```python
from build123d import *

# Parameters (mm, degrees)
F0_R     = 5.5
F0_R_2   = 8
F1_DEPTH = 6
F3_DEPTH = 25
F4_W     = 30
F4_H     = 6
F5_DEPTH = 25
F6_W     = 21
F6_H     = 7
F6_H_2   = 6
F7_DEPTH = 25


with BuildPart() as f1:
    # F0 (on Front) → F1 (new body)
    with BuildSketch(Plane.XZ):
        with BuildLine():
            Line((-59.436191, 0), (-59.436191, -101.490244))
            Line((-59.436191, -101.490244), (-19.436191, -101.490244))
            Line((-19.436191, -101.490244), (-19.436191, -78.490244))
            ThreePointArc((-19.436191, -78.490244), (-16.507259, -71.419176), (-9.436191, -68.490244))
            Line((-9.436191, -68.490244), (0.563809, -68.490244))
            ThreePointArc((0.563809, -68.490244), (7.634877, -65.561312), (10.563809, -58.490244))
            Line((10.563809, -58.490244), (10.563809, -53.490244))
            Line((10.563809, -53.490244), (10.563809, -48.490244))
            ThreePointArc((10.563809, -48.490244), (7.634877, -41.419176), (0.563809, -38.490244))
            Line((0.563809, -38.490244), (-4.436191, -38.490244))
            Line((-4.436191, -38.490244), (-9.436191, -38.490244))
            ThreePointArc((-9.436191, -38.490244), (-16.507259, -35.561312), (-19.436191, -28.490244))
            Line((-19.436191, -28.490244), (-19.436191, 3.509756))
            ThreePointArc((-19.436191, 3.509756), (-16.507259, 10.580824), (-9.436191, 13.509756))
            ThreePointArc((-9.436191, 13.509756), (-2.365123, 16.438688), (0.563809, 23.509756))
            Line((0.563809, 23.509756), (0.563809, 33.509756))
            Line((0.563809, 33.509756), (0.563809, 43.509756))
            ThreePointArc((0.563809, 43.509756), (-2.365123, 50.580824), (-9.436191, 53.509756))
            ThreePointArc((-9.436191, 53.509756), (-43.651687, 40.011908), (-59.436191, 6.789303))
            Line((-59.436191, 6.789303), (-59.436191, 0))
        make_face()
        with Locations((-4.436191, -53.490244)):
            Circle(F0_R, mode=Mode.SUBTRACT)
        with Locations((-19.436191, 33.509756)):
            Circle(F0_R_2, mode=Mode.SUBTRACT)
    extrude(amount=F1_DEPTH)

    # F2 (on face) → F3 (cut)
    with BuildSketch(Plane.XZ.offset(6)):
        with BuildLine():
            Line((-59.436191, 6.789303), (-59.436191, -101.490244))
            Line((-59.436191, -101.490244), (-49.436191, -101.490244))
            Line((-49.436191, -101.490244), (-49.436191, 33.586102))
            ThreePointArc((-49.436191, 33.586102), (-56.388476, 20.916254), (-59.436191, 6.789303))
        make_face()
    extrude(amount=-F3_DEPTH, mode=Mode.SUBTRACT)

    # F4 (on face) → F5 (cut)
    with BuildSketch(Plane.XZ.offset(6)):
        with Locations((-34.436191, -98.490244)):
            Rectangle(F4_W, F4_H)
    extrude(amount=-F5_DEPTH, mode=Mode.SUBTRACT)

    # F6 (on face) → F7 (cut)
    with BuildSketch(Plane.XZ.offset(6)):
        with Locations((-34.436191, -45.490244)):
            Rectangle(F6_W, F6_H)
        with Locations((-34.436191, 9.509756)):
            Rectangle(F6_W, F6_H_2)
    extrude(amount=-F7_DEPTH, mode=Mode.SUBTRACT)


solid = f1.part
```
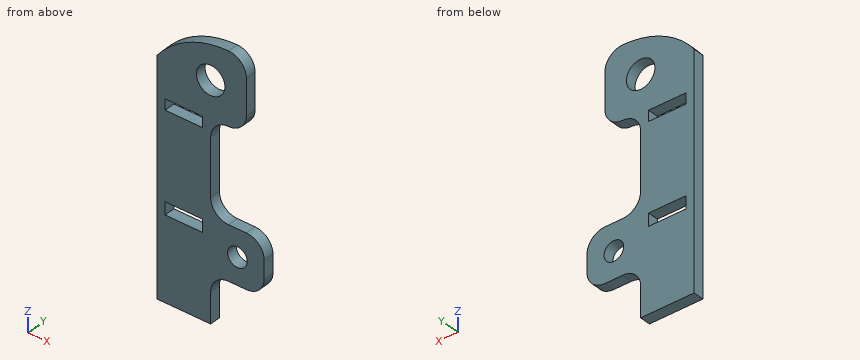
CAD build for the part. Positions are in the model's coordinates, mm. Round coordinates to 2 decimals unless told otherwise and drop trailing zeros. Loops run counter-clockwise (first coordinate to the right, second up) from the corner with the lowest first, then second, coordinate; pieces in that order, holes last. Notation, with made-up numbers: M 81.25,-10 L 115.25,-10 A33 cw 115.25,29 Z; hole C 74.5,17.5 d3. An arc over 180 degrees is marked long. Return JSON: item names as keys, results as strings. Group by question number.
(1) Saw through at B-B, the plane x = -6.5. List the corners of the cut face in (y, z).
(2) Saw through at C-C, the plane y = -5.1. List the corners of the cut face in (x, z), and give its area (3 significant figures).
(3) Drop flat-ended pins along their axis: P1, Ø1.8, axis at y = -3, z = 29.5, coming from the +X side; P2, Ø3, axis at y = -2.5, z = -85.5, coming from the +X side; P3, Ø3, axis at x = -23, y = -1.5, coming from the +Z side. Give the stop position or say it passes through.
(4) Saw through at A-A, the plane z = -46.5. List the corners of the cut face in (x, y), and give its area (3 significant figures).
(5) Wall check: probe 1 along Z at (x, y) = (-24.5, -1.4); probe 2 along Z at (x, y) = (-35, -0.3); probe 3 along Z at (x, y) = (-25, -2.7). Give the ranges that are in metal, low to high. Write a range as [from, to].
(6) Saw through at D-D, the plane x = -32. List the corners of the cut face in (y, z).
Answer list:
{
 "1": {"outline": "M -6,-68.49 L 0,-68.49 L 0,-58.59 L -6,-58.59 Z; M -6,-48.39 L 0,-48.39 L 0,-38.49 L -6,-38.49 Z; M -6,13.95 L 0,13.95 L 0,53.07 L -6,53.07 Z"},
 "2": {"outline": "M -49.44,-95.49 L -19.44,-95.49 L -19.44,-78.49 A10 cw -9.44,-68.49 L 0.56,-68.49 A10 ccw 10.56,-58.49 L 10.56,-48.49 A10 ccw 0.56,-38.49 L -9.44,-38.49 A10 cw -19.44,-28.49 L -19.44,3.51 A10 cw -9.44,13.51 A10 ccw 0.56,23.51 L 0.56,43.51 A10 ccw -9.44,53.51 A50.12 ccw -49.44,33.59 Z; hole M -44.94,-48.99 L -23.94,-48.99 L -23.94,-41.99 L -44.94,-41.99 Z; hole M -44.94,6.51 L -23.94,6.51 L -23.94,12.51 L -44.94,12.51 Z; hole C -19.44,33.51 d16; hole C -4.44,-53.49 d11", "area": "5,340 mm2"},
 "3": {"P1": "x = 0.56", "P2": "x = -19.44", "P3": "z = 52.04"},
 "4": {"outline": "M -49.44,-6 L -44.94,-6 L -44.94,0 L -49.44,0 Z; M -23.94,-6 L 10.36,-6 L 10.36,0 L -23.94,0 Z", "area": "233 mm2"},
 "5": {"probe 1": "[-95.49, -48.99], [-41.99, 6.51], [12.51, 27.32], [39.7, 51.19]", "probe 2": "[-95.49, -48.99], [-41.99, 6.51], [12.51, 46.5]", "probe 3": "[-95.49, -48.99], [-41.99, 6.51], [12.51, 27.76], [39.26, 51.03]"},
 "6": {"outline": "M -6,-95.49 L 0,-95.49 L 0,-48.99 L -6,-48.99 Z; M -6,-41.99 L 0,-41.99 L 0,6.51 L -6,6.51 Z; M -6,12.51 L 0,12.51 L 0,48.14 L -6,48.14 Z"}
}
